Can you work these out from the model? Positions are in its coordinate system, mm. A direction names the side the tool comes from. Round coordinates to 2 decimals unless told otherwise and drop trailing zeros. Loops run counter-clockwise (first coordinate to the right, second up) from the corner with the lowest first, then second, coordinate; pieces in that order, holes last. Notation, with made-up numbers: (66.25, 22) -> (70.25, 22) arc R22 cw to (70.25, 45) -> close; hole circle Ø8 at (26, -11.5). An arc over 180 degrees is marked (long way). Answer as a JSON object with one key per item and string values.
```python
from build123d import *

# Parameters (mm, degrees)
F0_W     = 31.75
F0_H     = 7.9375
F1_DEPTH = 9.525
F2_R     = 2.4257
F3_DEPTH = 1.778
F5_W     = 29.5656
F5_H     = 5.7531
F6_DEPTH = 8.4328


with BuildPart() as f1:
    # F0 (on Top) → F1 (new body)
    with BuildSketch(Plane.XY):
        with Locations((-14.812947, 15.498804)):
            Rectangle(F0_W, F0_H)
    extrude(amount=F1_DEPTH)

    # F2 (on face) → F3 (join)
    with BuildSketch(Plane.XY.offset(9.525)):
        with Locations((-26.852553, 15.505154)):
            Circle(F2_R)
        with Locations((-18.826153, 15.505154)):
            Circle(F2_R)
        with Locations((-10.799753, 15.517854)):
            Circle(F2_R)
        with Locations((-2.773347, 15.505154)):
            Circle(F2_R)
    extrude(amount=F3_DEPTH)

    # F5 (on face) → F6 (cut)
    with BuildSketch(Plane(origin=(0, 0, 0), x_dir=(1, 0, 0), z_dir=(0, 0, -1))):
        with Locations((-14.812947, -15.498804)):
            Rectangle(F5_W, F5_H)
    extrude(amount=-F6_DEPTH, mode=Mode.SUBTRACT)


solid = f1.part
```
Q1. We'd pull the mould along X, two halves only. Please class faces 4 (the flat face through (1.062, 15, 5)), 5 (the cylindrical face through (-21.25, 15.61, 10.4)), 6 (the flat face through (-11, 16, 11.303)): pulls with the +X half, pulls with the -X half, needs draft (parallel to the pull), parting line crosses it, or undercut.
Determined:
{"face 4": "pulls with the +X half", "face 5": "undercut", "face 6": "needs draft"}
Q2. I want a section at C-C, the plane y = 14. Write out the boundary of the cut face in (x, z) (3 decimals).
Determined:
{"outline": "(-30.688, 0) -> (-29.596, 0) -> (-29.596, 8.433) -> (-0.03, 8.433) -> (-0.03, 0) -> (1.062, 0) -> (1.062, 9.525) -> (-0.871, 9.525) -> (-0.871, 11.303) -> (-4.676, 11.303) -> (-4.676, 9.525) -> (-8.908, 9.525) -> (-8.908, 11.303) -> (-12.692, 11.303) -> (-12.692, 9.525) -> (-16.924, 9.525) -> (-16.924, 11.303) -> (-20.728, 11.303) -> (-20.728, 9.525) -> (-24.95, 9.525) -> (-24.95, 11.303) -> (-28.755, 11.303) -> (-28.755, 9.525) -> (-30.688, 9.525) -> close"}
Q3. I'm going to push flat-ended pins straight in: pin 1 (3 mm diameter, centred on x = -15.5, y = 13, fed in from +Z) (3 decimals); pin 2 (1.7 mm diameter, centred on x = -15.5, y = 16.5, fed in from -Z). Where does each tip first touch, or does it pass through?
Determined:
{"pin 1": "z = 9.525", "pin 2": "z = 8.43"}
Q4. I want a section at D-D, the plane z = 10.5. Write out the boundary of the cut face in (x, y).
Determined:
{"outline": "circle Ø4.85 at (-26.85, 15.51); circle Ø4.85 at (-18.83, 15.51); circle Ø4.85 at (-10.8, 15.52); circle Ø4.85 at (-2.77, 15.51)"}
Q5. I want a section at B-B, the plane x = -16. Write out the boundary of the cut face in (y, z) (3 decimals), then the cut area to 3 significant figures.
Determined:
{"outline": "(11.53, 0) -> (12.622, 0) -> (12.622, 8.433) -> (18.375, 8.433) -> (18.375, 0) -> (19.468, 0) -> (19.468, 9.525) -> (11.53, 9.525) -> close", "area": "27.1 mm²"}
Q6. If I drill on L1, parallel to X at y = 13.5, z = 7.75; L2, parallel to Y at x = -27, z = 3.75; L3, parallel to X at y = 17, z = 10.25, over which ranges is the centre line in solid material (lowest first)? Write a range as [from, to].
Determined:
{"L1": "[-30.69, -29.6], [-0.03, 1.06]", "L2": "[11.53, 12.62], [18.38, 19.47]", "L3": "[-28.76, -24.94], [-20.74, -16.92], [-12.72, -8.88], [-4.68, -0.86]"}
Q7. I want a section at A-A, the plane z = 5. Write out the boundary of the cut face in (x, y), then the cut area to 3 significant figures.
Determined:
{"outline": "(-30.69, 11.53) -> (1.06, 11.53) -> (1.06, 19.47) -> (-30.69, 19.47) -> close; hole (-29.6, 12.62) -> (-0.03, 12.62) -> (-0.03, 18.38) -> (-29.6, 18.38) -> close", "area": "81.9 mm²"}
Q8. On a 3-axis mill with a long thin cutter (end or side, diameter ignored), from which of +Z, -Z, +X, -X, +Y, -Y can I reach the whole of each face in a straight line? I mean faces 1 (the cylindrical face through (-12.725, 14.042, 10.402)), 2 (the flat face through (-29.596, 16, 4)), 3 (the flat face through (-19, 16, 11.303)). Say none if no direction works.
Determined:
{"face 1": "+Z", "face 2": "-Z", "face 3": "+Z, +X, -X, +Y, -Y"}
